```python
from build123d import *

# Parameters (mm, degrees)
BOSS_EXTRUDE1_DEPTH = 15
SKETCH3_R           = 2.45
BOSS_EXTRUDE2_DEPTH = 12.5
FILLET2_R           = 10
SKETCH8_R           = 1.6
CUT_EXTRUDE6_DEPTH  = 29.681007074
CUT_EXTRUDE7_REACH  = 30.681
SKETCH9_W           = 7.5
SKETCH9_H           = 10
CUT_EXTRUDE8_REACH  = 30.681
SKETCH10_R          = 1.6
FILLET3_R           = 1
FILLET4_R           = 2


with BuildPart() as part:
    # Sketch2 → Boss-Extrude1 (new body)
    with BuildSketch(Plane.XY):
        with BuildLine():
            Line((-2.5, -6.008335649), (-2.5, -21.008335649))
            Line((-2.5, -21.008335649), (-5, -21.008335649))
            Line((-5, -21.008335649), (-5, -6.008335649))
            Line((-5, -6.008335649), (-5, -5.590169944))
            ThreePointArc((-5, -5.590169944), (0, 7.5), (5, -5.590169944))
            Line((5, -5.590169944), (5, -6.008335649))
            Line((5, -6.008335649), (5, -21.008335649))
            Line((5, -21.008335649), (2.5, -21.008335649))
            Line((2.5, -21.008335649), (2.5, -6.008335649))
            Line((2.5, -6.008335649), (-2.5, -6.008335649))
        make_face()
    extrude(amount=BOSS_EXTRUDE1_DEPTH)

    # Sketch3 → Boss-Extrude2 (add)
    with BuildSketch(Plane(origin=(0, 0, 0), x_dir=(-1, 0, 0), z_dir=(0, 0, -1))):
        Circle(SKETCH3_R)
    extrude(amount=BOSS_EXTRUDE2_DEPTH)

    # Fillet2
    fillet2_edges = [part.edges().sort_by_distance(p)[0] for p in [
        (-5, -5.590169944, 7.5),
        (5, -5.590169944, 7.5),
    ]]
    fillet(fillet2_edges, radius=FILLET2_R)

    # Sketch8 → Cut-Extrude6 (cut, through all)
    with BuildSketch(Plane(origin=(5, 0, 0), x_dir=(0, 0, -1), z_dir=(1, 0, 0))):
        with Locations((-3.5, -16.008335649)):
            Circle(SKETCH8_R)
    extrude(amount=-CUT_EXTRUDE6_DEPTH, mode=Mode.SUBTRACT)

    # Sketch9 → Cut-Extrude7 (cut, up to next)
    with BuildSketch(Plane.ZY.offset(5), mode=Mode.PRIVATE) as cut_extrude7_sk1:
        with Locations((11.25, -16.008335649)):
            Rectangle(SKETCH9_W, SKETCH9_H)
    cut_extrude7_tool1 = extrude(cut_extrude7_sk1.sketch, amount=-CUT_EXTRUDE7_REACH, mode=Mode.PRIVATE) & part.part
    add(cut_extrude7_tool1.solids().sort_by_distance((-5, -16.008336, 11.25))[0], mode=Mode.SUBTRACT)

    # Sketch10 → Cut-Extrude8 (cut, up to next)
    with BuildSketch(Plane(origin=(5, 0, 0), x_dir=(0, 0, -1), z_dir=(1, 0, 0)), mode=Mode.PRIVATE) as cut_extrude8_sk1:
        with Locations((-11.5, -16.008335649)):
            Circle(SKETCH10_R)
    cut_extrude8_tool1 = extrude(cut_extrude8_sk1.sketch, amount=-CUT_EXTRUDE8_REACH, mode=Mode.PRIVATE) & part.part
    add(cut_extrude8_tool1.solids().sort_by_distance((5, -16.008336, 11.5))[0], mode=Mode.SUBTRACT)

    # Fillet3
    fillet3_edges = [part.edges().sort_by_distance(p)[0] for p in [
        (2.45, 0, 0),
    ]]
    fillet(fillet3_edges, radius=FILLET3_R)

    # Fillet4
    fillet4_edges = [part.edges().sort_by_distance(p)[0] for p in [
        (2.5, -6.008335649, 7.5),
        (-2.5, -6.008335649, 7.5),
        (-3.75, -11.008335649, 7.5),
        (-3.75, -11.008335649, 15),
        (-2.5, -21.008335649, 3.75),
        (2.5, -21.008335649, 7.5),
    ]]
    fillet(fillet4_edges, radius=FILLET4_R)


solid = part.part
```
The model under review builds one solid part; all positions refer to its coordinate system, in mm. A direction names the side the tool comes from. Give positions to 0.01 mm unless a question says otherwise; leave off trailing zeros. Order: outer loops, then holes, each group sorted by start corner. A loop starts at its lowest first (then second) coordinate and runs counter-clockwise, first axis right, second up. Notation, with made-up numbers: (14, 60.5) - (30, 60.5) arc R16 ccw to (30, 65.5) - close; hole circle Ø10 at (67, 2.5). An arc over 180 degrees is marked (long way). Use CSV: the item, a comma, the result in double quotes. Start each with the question number.
Q1. We need section D-D, the plane z = 11. Write out the cut boundary in (x, y).
Q2. Clearance check with flat-ended pins moving along their axes: pin 1 Ø10 at (y, z) = (-10.5, 7) entering from +X; pin 2 Ø0.5 at (x, z) = (0, 9) entering from -Y; pin 3 Ø1.9 at (y, z) = (-16.01, 11.5) entering from +X; pin 4 Ø13 at (y, z) = (-14.5, 7.5) entering from -X. State where each tip first meets the part, or that it passes through.
Q3. We need section A-A, the plane z = 3.5. Write out the cut boundary in (x, y).
Q4. Tool access review of faces 5 (the cylindrical face through (0.5, -2.4, -6.7)), 6 (the cylindrical face through (5.374, -6.305, 7.605)), 7 (the flat face through (-5, -15, 6)), 8 (the cylindrical face through (3.07, -20.407, 7.605)), 9 (the flat face through (-4, -11.008, 11)): name each direction out of +Z, -Z, +X, -X, +Y, -Y from which nothing blocks a thin tool from reaching the whole face with its end or side.
Q5. The part is to be moulded in two halves that separate along Z. For faces 1 (the cylindrical face through (-3.732, -14.422, 3.708)), 2 (the cylindrical face through (3.768, -14.422, 3.708)), 3 (the flat face through (-2, -3, 0)), 4 (the cylindrical face through (-3.101, -20.438, 3.802)), say which applies: +Z half, -Z half, draft (parallel to the pull), parting line (faces both ways), or undercut.
Q6. We need section C-C, the plane x = 0. Write out the cut boundary in (y, z).
Q7. We need section B-B, the plane y = -8.5. Write out the cut boundary in (x, z).
Q8. To check wall thickness, follow line 1 along X through (y, z) = (-9.5, 13); line 2 along Z through (x, y) = (4.75, 3.75); line 3 along Z through (x, y) = (-2.75, -16.25). State the ranges of each line that lie inside material, in increasing order. Write a range as [from, to].
Outcome:
1,outline,"(-6.43, -3.86) arc R10 cw to (-5, -9.01) - (-5, -11.01) - (-2.5, -11.01) - (-2.5, -8.01) arc R2 cw to (-0.5, -6.01) - (0.5, -6.01) arc R2 cw to (2.5, -8.01) - (2.5, -14.49) - (5, -14.49) - (5, -9.01) arc R10 cw to (6.43, -3.86) arc R7.5 ccw (long way) to start; (2.5, -19.01) arc R2 ccw to (4.5, -21.01) - (5, -21.01) - (5, -17.53) - (2.5, -17.53) - close"
2,pin 1,"stops at x = 5.64"
2,pin 2,"stops at y = -6.01"
2,pin 3,"passes through"
2,pin 4,"stops at x = -5.05"
3,outline,"(-6.43, -3.86) arc R10 cw to (-5, -9.01) - (-5, -14.41) - (-2.5, -14.41) - (-2.5, -8.01) arc R2 cw to (-0.5, -6.01) - (0.5, -6.01) arc R2 cw to (2.5, -8.01) - (2.5, -14.41) - (5, -14.41) - (5, -9.01) arc R10 cw to (6.43, -3.86) arc R7.5 ccw (long way) to start; (-5, -21.01) - (-4.5, -21.01) arc R2 ccw to (-2.5, -19.01) - (-2.5, -17.61) - (-5, -17.61) - close; (2.5, -19.01) arc R2 ccw to (4.5, -21.01) - (5, -21.01) - (5, -17.61) - (2.5, -17.61) - close"
4,face 5,"-Z"
4,face 6,"+Z, -Z, +X, -Y"
4,face 7,"+Z, -Z, -X, -Y"
4,face 8,"+Z, -Z, -Y"
4,face 9,"+Z, -X, -Y"
5,face 1,"undercut"
5,face 2,"undercut"
5,face 3,"-Z half"
5,face 4,"draft"
6,outline,"(-6.01, 0) - (-3.45, 0) arc R1 cw to (-2.45, -1) - (-2.45, -12.5) - (2.45, -12.5) - (2.45, -1) arc R1 cw to (3.45, 0) - (7.5, 0) - (7.5, 15) - (-6.01, 15) - close"
7,outline,"(-5.01, 0) - (-2.5, 0) - (-2.5, 15) - (-5.01, 15) - close; (2.5, 0) - (5.01, 0) - (5.01, 15) - (2.5, 15) - close"
8,line 1,"x = [-5, -2.5], [2.5, 5]"
8,line 2,"z = [0, 15]"
8,line 3,"z = [0, 1.92], [5.08, 7.5]"
